from build123d import *

# Parameters (mm, degrees)
BOSS_EXTRUDE1_DEPTH                          = 25.4
SKETCH2_W                                    = 234.95
SKETCH2_H                                    = 139.7
CUT_EXTRUDE1_DEPTH                           = 51.8
EXTRUDE_THIN1_DEPTH                          = 50.8
EXTRUDE_THIN2_DEPTH                          = 50.8
FILLET5_R                                    = 3.175
SKETCH11_W                                   = 33.02
SKETCH11_H                                   = 38.1
BOSS_EXTRUDE2_DEPTH                          = 50.8
TAPPED_HOLE_FOR_3_8_16_HELICOIL1_D           = 10.0838
TAPPED_HOLE_FOR_3_8_16_HELICOIL1_DEPTH       = 29.21
TAPPED_HOLE_FOR_3_8_16_HELICOIL1_CSINK_D     = 12.95908
TAPPED_HOLE_FOR_3_8_16_HELICOIL1_CSINK_ANGLE = 90
TAPPED_HOLE_FOR_3_8_16_HELICOIL1_TIP         = 3.029479155
CUT_EXTRUDE2_DEPTH                           = 51.8
FILLET1_R                                    = 3.175
FILLET2_R                                    = 1.5875
FILLET3_R                                    = 9.525
F_1_2_CLEARANCE_HOLE1_AT_2_COUNT             = 2
F_1_2_CLEARANCE_HOLE1_AT_2_PITCH             = 225.425


with BuildPart() as part:
    # Sketch1 → Boss-Extrude1 (new body, symmetric)
    with BuildSketch(Plane(origin=(0, 0, 0), x_dir=(0, 0, -1), z_dir=(1, 0, 0))):
        Polygon((311.15, -88.9), (19.05, -88.9), (19.05, -139.7), (0, -139.7), (0, 127), (19.05, 127), (19.05, 76.2), (260.35, 76.2), (260.35, -76.2), (311.15, -76.2), align=None)
    extrude(amount=BOSS_EXTRUDE1_DEPTH, both=True)

    # Sketch2 → Cut-Extrude1 (cut, through all)
    with BuildSketch(Plane.ZY.offset(25.4)):
        with Locations((-130.175, -6.35)):
            Rectangle(SKETCH2_W, SKETCH2_H)
    extrude(amount=-CUT_EXTRUDE1_DEPTH, mode=Mode.SUBTRACT)

    # Sketch3 → Extrude-Thin1 (add)
    with BuildSketch(Plane.ZY.offset(25.4)):
        Polygon((-250.895328745, 58.041947111), (-15.945328745, -81.658052889), (-9.454671255, -70.741947111), (-244.404671255, 68.958052889), align=None)
    extrude(amount=-EXTRUDE_THIN1_DEPTH)

    # Sketch4 → Extrude-Thin2 (add)
    with BuildSketch(Plane.ZY.offset(25.4)):
        Polygon((-244.404671255, -81.658052889), (-9.454671255, 58.041947111), (-15.945328745, 68.958052889), (-250.895328745, -70.741947111), align=None)
    extrude(amount=-EXTRUDE_THIN2_DEPTH)

    # Fillet5
    fillet5_edges = [part.edges().sort_by_distance(p)[0] for p in [
        (0, -76.2, -235.225218669),
        (0, 63.5, -235.225218669),
    ]]
    fillet(fillet5_edges, radius=FILLET5_R)

    # Sketch11 → Boss-Extrude2 (add)
    with BuildSketch(Plane.ZY.offset(25.4)):
        with Locations((-243.84, -57.15)):
            Rectangle(SKETCH11_W, SKETCH11_H)
    boss_extrude2 = extrude(amount=-BOSS_EXTRUDE2_DEPTH)

    # Mirror2: Boss-Extrude2 across plane
    add(boss_extrude2.mirror(Plane.ZX))

    # Tapped Hole for 3/8-16 Helicoil1
    with Locations(Plane(origin=(-14.876894715, 2.702023936, -260.35), x_dir=(-1, 0, 0), z_dir=(0, 0, -1))):
        with Locations((-14.876894715, 54.447976064), (-14.876894715, -59.852023936)):
            CounterSinkHole(TAPPED_HOLE_FOR_3_8_16_HELICOIL1_D / 2, TAPPED_HOLE_FOR_3_8_16_HELICOIL1_CSINK_D / 2, depth=TAPPED_HOLE_FOR_3_8_16_HELICOIL1_DEPTH, counter_sink_angle=TAPPED_HOLE_FOR_3_8_16_HELICOIL1_CSINK_ANGLE)
            with Locations((0, 0, -(TAPPED_HOLE_FOR_3_8_16_HELICOIL1_DEPTH + TAPPED_HOLE_FOR_3_8_16_HELICOIL1_TIP / 2))):  # 118° drill point
                Cone(0, TAPPED_HOLE_FOR_3_8_16_HELICOIL1_D / 2, TAPPED_HOLE_FOR_3_8_16_HELICOIL1_TIP, mode=Mode.SUBTRACT)

    # Sketch12 → Cut-Extrude2 (cut, through all)
    with BuildSketch(Plane.ZY.offset(25.4)):
        with BuildLine():
            Line((-260.35, -76.2), (-260.35, -69.85))
            ThreePointArc((-260.35, -69.85), (-257.175, -73.025), (-260.35, -76.2))
        make_face()
    extrude(amount=-CUT_EXTRUDE2_DEPTH, mode=Mode.SUBTRACT)

    # Fillet1
    fillet1_edges = [part.edges().sort_by_distance(p)[0] for p in [
        (0, -56.73013002, -227.33),
        (0, -38.1, -247.65),
        (0, 44.03013002, -227.33),
        (0, 38.1, -247.65),
        (0, -76.2, -25.124781331),
        (0, -68.812292182, -12.7),
        (0, -6.35, -142.599781331),
        (0, -13.737707818, -130.175),
        (0, 56.112292182, -12.7),
        (0, 63.5, -25.124781331),
        (0, 1.037707818, -130.175),
    ]]
    fillet(fillet1_edges, radius=FILLET1_R)

    # Fillet2
    fillet2_edges = [part.edges().sort_by_distance(p)[0] for p in [
        (0, 127, 0),
        (0, 127, -19.05),
        (0, -139.7, 0),
        (0, -139.7, -19.05),
        (0, -88.9, -311.15),
        (0, -76.2, -311.15),
        (0, 76.2, -260.35),
        (0, 38.1, -227.33),
        (0, -38.1, -227.33),
        (0, -69.85, -260.35),
    ]]
    fillet(fillet2_edges, radius=FILLET2_R)

    # Fillet3
    fillet3_edges = [part.edges().sort_by_distance(p)[0] for p in [
        (0, -88.9, -19.05),
        (0, 76.2, -19.05),
    ]]
    fillet(fillet3_edges, radius=FILLET3_R)

    # Sketch9 → 1/2 Clearance Hole1 (revolve, cut)
    with BuildSketch(Plane(origin=(0, 106.3625, -19.05), x_dir=(0, 1, 0), z_dir=(1, 0, 0))):
        Polygon((0, 0), (0, 19.05), (7.58063, 19.05), (6.94563, 18.415), (6.94563, 0.635), (7.58063, 0), align=None)
    f_1_2_clearance_hole1 = revolve(axis=Axis((0, 106.3625, -25.4), (0, 0, 1)), mode=Mode.SUBTRACT)

    # 1/2 Clearance Hole1 at 2: 1/2 Clearance Hole1 ×2
    with Locations(*[(0, -i * F_1_2_CLEARANCE_HOLE1_AT_2_PITCH, 0) for i in range(1, F_1_2_CLEARANCE_HOLE1_AT_2_COUNT)]):
        add(f_1_2_clearance_hole1, mode=Mode.SUBTRACT)


solid = part.part
Verification items for the finished model (mm, model axes). A direction names the side the tool comes from. Coordinates: 2 decimals unless noted, no trailing zeros. Write each loop counter-clockwise with the first axis right and the second up, starting at its lowest first coordinate (ties: lowest second). Pieces come first, ordered by that corner, then holes. Notation, with made-up numbers: M 87,27 L 123,27 A23 cw 123,38 Z; hole C -16,74 d10. An arc over 180 degrees is marked long. Use CSV: the item, a comma, the result in double quotes.
Q1. Mould release check, pull along Y, two halves, no side actions. Record for faces 1 (the cylindrical face through (-1.093, 52.228, -244.832)), 2 (the flat face through (-25.4, -6, -145)), 3 (the flat face through (0, 127, -9)): pulls with the +Y half, pulls with the -Y half, needs draft (parallel to the pull), parting line crosses it, or undercut.
Computed values:
face 1,"undercut"
face 2,"needs draft"
face 3,"pulls with the +Y half"
Q2. Section check A-A, the plane z = -105. Enter the section's corners in (x, y), and give its area (3 significant figures).
Computed values:
outline,"M -25.4,-88.9 L 25.4,-88.9 L 25.4,-76.2 L -25.4,-76.2 Z; M -25.4,-28.71 L 25.4,-28.71 L 25.4,-13.93 L -25.4,-13.93 Z; M -25.4,1.23 L 25.4,1.23 L 25.4,16.01 L -25.4,16.01 Z; M -25.4,63.5 L 25.4,63.5 L 25.4,76.2 L -25.4,76.2 Z"
area,"2,790 mm²"
Q3. Section check D-D, the plane y = -107.5. Enter the section's corners in (x, z), and give its area (3 significant figures).
Computed values:
outline,"M -25.4,-19.05 L 25.4,-19.05 L 25.4,0 L -25.4,0 Z"
area,"968 mm²"
Q4. Section check B-B, the plane y = 23. Enter the section's corners in (x, z).
Computed values:
outline,"M -25.4,-260.35 L 25.4,-260.35 L 25.4,-247.65 L -25.4,-247.65 Z; M -25.4,-191.96 L 25.4,-191.96 L 25.4,-167.11 L -25.4,-167.11 Z; M -25.4,-93.24 L 25.4,-93.24 L 25.4,-68.39 L -25.4,-68.39 Z; M -25.4,-12.7 L 25.4,-12.7 L 25.4,0 L -25.4,0 Z"
Q5. Set-up check for faces 4 (the cylindrical face through (-0.36, -91.62, -21.91)), 5 (the flat face through (0, -76.2, -285)), 6 (the cylindrical face through (2.71, -52.9, -244.83)), 7 (the cylindrical face through (4.226, 100.851, -9.649)), 8 (the flat face through (-0.36, 30.19, -81.15)): record each of +Z, -Z, +X, -X, +Y, -Y from which the full face is reachable in a straight line by a thin tool's end or side.
Computed values:
face 4,"-Z, +X, -X, -Y"
face 5,"-Z, +X, -X, +Y"
face 6,"-Z"
face 7,"+Z, -Z"
face 8,"+X, -X"
Q6. Thickness scan on line 1 along Y through (x, z) = (0, -249.25); line 2 along Y through (x, z) = (0, -8); line 3 along Y through (x, z) = (0, -240). Record the ranges inside material, lowest first. Write a range as [from, to].
Computed values:
line 1,"[-88.9, -62.19], [-52.11, 52.11], [62.19, 76.2]"
line 2,"[-139.7, -126.01], [-112.12, 99.42], [113.31, 127]"
line 3,"[-88.9, -62.19], [-52.11, -38.1], [38.1, 52.11], [62.19, 76.2]"
Q7. Section check C-C, the plane x = 18. State how many separate pieces and enclosed holes the cut face has, and give its area (3 significant figures).
Computed values:
separate pieces,"1"
enclosed holes,"4"
area,"20,200 mm²"
Q8. Go/stop test with flat-tipped pins: P1, Ø1, axis at x = 18, y = -1, coming from the -Z side; P2, Ø12, axis at x = 13, y = -102, coming from the -Z side; P3, Ø11.5, axis at x = 0, y = -57.15, coming from the +Z side; P4, Ø8, axis at x = 11, z = -233, coming from the -Y side. Record where each tip stops, or that it passes through.
Computed values:
P1,"z = -260.35"
P2,"z = -19.36"
P3,"z = 0"
P4,"y = -88.9"
